The listing builds one solid part. Answer for the finished solid, in the listing's coordinates (mm). Face numbers are marked on the shaded views. A direction names the side the tool comes from. Round coordinates to 2 decimals unless told otherwise and drop trailing zeros. Write each loop counter-clockwise with the first axis right and the second up, starting at its lowest first coordinate (ties: lowest second). Pieces come first, ordered by that corner, then holes. Notation, with made-up numbers: (83, 12) - (132, 12) arc R19 ccw to (132, 17) - close; hole circle Ø11 at (-16.5, 70.25). An arc over 180 degrees is marked (long way). Use a Markdown table: item, result. Add a question column.
1) Each of these flat-tipped pins is pushed along its axis until it touches: P1, Ø1.5, axis at x = 16.5, z = 14.5, coming from the +Y side; P2, Ø12.5, axis at x = 43, z = 21.5, coming from the -Y side; P3, Ø3, axis at y = 34, z = 10.5, coming from the +X side; P4, Ø6, axis at y = 27, z = 7, coming from the -X side. Where does it stop, or does it pass through?
2) A cutting plane is placed at A-A (x = 8.7). Give the vertices of the cut face in (y, z), then the cut area to 3 significant figures.
3) A tool of negligible diameter and unlimited length cuts with its end or side. For the marked faces 1, 2 and 3, from which of +Z, -Z, +X, -X, +Y, -Y can it reach the whole face along a straight path? Write none if from no direction.
4) Find the intervals of material crossed by probe 1 along X at (y, z) = (1.2, 21.5); probe 2 along Y at (x, z) = (26, 30.5); probe 3 along Z at (x, y) = (25.5, 9.5), in increasing order. Write a range as from..to.
5) A cutting plane is placed at D-D (z = 38.5). Give the vertices of the cut face in (x, y), then the cut area to 3 significant figures.
6) A cutting plane is placed at C-C (y = 139.5). Give the vertices of the cut face in (x, z), then the cut area to 3 significant figures.
7) A cutting plane is placed at B-B (z = 24). Give the vertices of the cut face in (x, y), then the cut area to 3 significant figures.
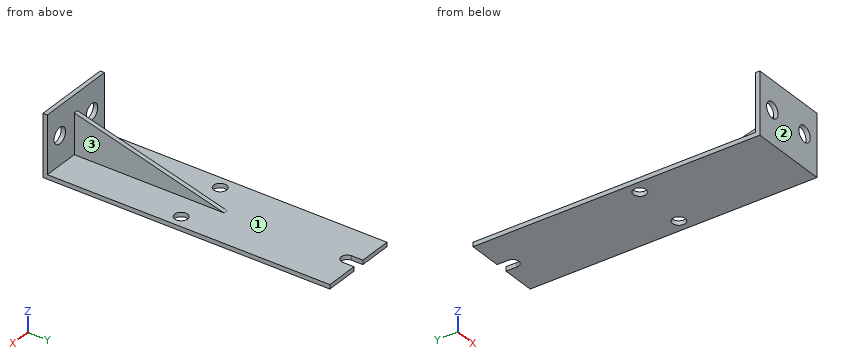
```python
from build123d import *

# Parameters (mm, degrees)
SZKIC1_W                    = 55
SZKIC1_H                    = 200
DODANIE_WYCI_GNI_CIE1_DEPTH = 1.5
SZKIC2_W                    = 55
SZKIC2_H                    = 3
DODANIE_WYCI_GNI_CIE2_DEPTH = 40
SZKIC3_R                    = 5.5
WYTNIJ_WYCI_GNI_CIE1_DEPTH  = 20
DODANIE_WYCI_GNI_CIE3_DEPTH = 1.5
SZKIC5_R                    = 4.5
WYTNIJ_WYCI_GNI_CIE3_DEPTH  = 212.834841327


with BuildPart() as part:
    # Szkic1 → Dodanie-wyci_gni_cie1 (new, symmetric)
    with BuildSketch(Plane.XY):
        with Locations((27.5, 100)):
            Rectangle(SZKIC1_W, SZKIC1_H)
    extrude(amount=DODANIE_WYCI_GNI_CIE1_DEPTH, both=True)



with BuildPart() as body_2:
    # Szkic2 → Dodanie-wyci_gni_cie2 (new body)
    with BuildSketch(Plane.XY.offset(1.5)):
        with Locations((27.5, 1.5)):
            Rectangle(SZKIC2_W, SZKIC2_H)
    extrude(amount=DODANIE_WYCI_GNI_CIE2_DEPTH)

    # Szkic3 → Wytnij-wyci_gni_cie1 (cut)
    with BuildSketch(Plane(origin=(0, 3, 0), x_dir=(1, 0, 0), z_dir=(0, 1, 0))):
        with Locations(Location((12, -21.5, 0), (0, 0, 270))):
            Circle(SZKIC3_R)
        with Locations(Location((43, -21.5, 0), (0, 0, 270))):
            Circle(SZKIC3_R)
    extrude(amount=-WYTNIJ_WYCI_GNI_CIE1_DEPTH, mode=Mode.SUBTRACT)


with BuildPart() as part_1:
    add(part.part)

    add(body_2.part)  # Dodanie-wyci_gni_cie3 merges body 2
    # Szkic4 → Dodanie-wyci_gni_cie3 (add, symmetric)
    with BuildSketch(Plane(origin=(27.5, 0, 0), x_dir=(0, 0, -1), z_dir=(1, 0, 0))):
        Polygon((-29.5, 3), (-1.5, 107.497422612), (-1.5, 3), align=None)
    extrude(amount=DODANIE_WYCI_GNI_CIE3_DEPTH, both=True)

    # Szkic5 → Wytnij-wyci_gni_cie3 (cut, through all)
    with BuildSketch(Plane(origin=(0, 0, -1.5), x_dir=(-1, 0, 0), z_dir=(0, 0, -1))):
        with Locations((-8.7, 90)):
            Circle(SZKIC5_R)
        with Locations((-46.3, 90)):
            Circle(SZKIC5_R)
        with BuildLine():
            Line((-31.75, 200), (-31.75, 192.25))
            ThreePointArc((-31.75, 192.25), (-27.5, 188), (-23.25, 192.25))
            Line((-23.25, 192.25), (-23.25, 200))
            Line((-23.25, 200), (-31.75, 200))
        make_face()
    extrude(amount=-WYTNIJ_WYCI_GNI_CIE3_DEPTH, mode=Mode.SUBTRACT)


solid = part_1.part
```
Entries:
| question | item | result |
|---|---|---|
| 1 | P1 | stops at y = 3 |
| 1 | P2 | stops at y = 0 |
| 1 | P3 | stops at x = 29 |
| 1 | P4 | stops at x = 26 |
| 2 | outline | (0, -1.5) - (85.5, -1.5) - (85.5, 1.5) - (3, 1.5) - (3, 17.1) - (0, 17.1) - close; (0, 25.9) - (3, 25.9) - (3, 41.5) - (0, 41.5) - close; (94.5, -1.5) - (200, -1.5) - (200, 1.5) - (94.5, 1.5) - close |
| 2 | area | 667 mm² |
| 3 | face 1 | +Z, +Y |
| 3 | face 2 | +Z, -Z, +X, -X, -Y |
| 3 | face 3 | +Z, +X, +Y |
| 4 | probe 1 | x = 0..6.5, 17.5..37.5, 48.5..55 |
| 4 | probe 2 | y = 0..3 |
| 4 | probe 3 | z = -1.5..1.5 |
| 5 | outline | (0, 0) - (55, 0) - (55, 3) - (0, 3) - close |
| 5 | area | 165 mm² |
| 6 | outline | (0, -1.5) - (55, -1.5) - (55, 1.5) - (0, 1.5) - close |
| 6 | area | 165 mm² |
| 7 | outline | (0, 0) - (7.1, 0) - (7.1, 3) - (0, 3) - close; (16.9, 0) - (38.1, 0) - (38.1, 3) - (29, 3) - (29, 23.53) - (26, 23.53) - (26, 3) - (16.9, 3) - close; (47.9, 0) - (55, 0) - (55, 3) - (47.9, 3) - close |
| 7 | area | 168 mm² |
